Input: dimensioned drawing with shaded views. Units: mm. Origin: part minimum x, y, z. A direction names the side the tool comes from. Round coordinates to 2 decimals unless told otherwise and drop trailing zeros. Loops run counter-clockwise (first coordinate to the right, second up) from the corner with the lowest first, then second, coordinate; pieces in that order, holes last. Notation, with made-up numbers: (19, 18.5) - (74, 18.5) arc R21 cw to (74, 43.5) - close; hole circle Ø10 at (48, -10.75). An arc over 180 degrees is marked (long way). Use CSV: the item, a comma, the result in double quotes. Start each with the question number.
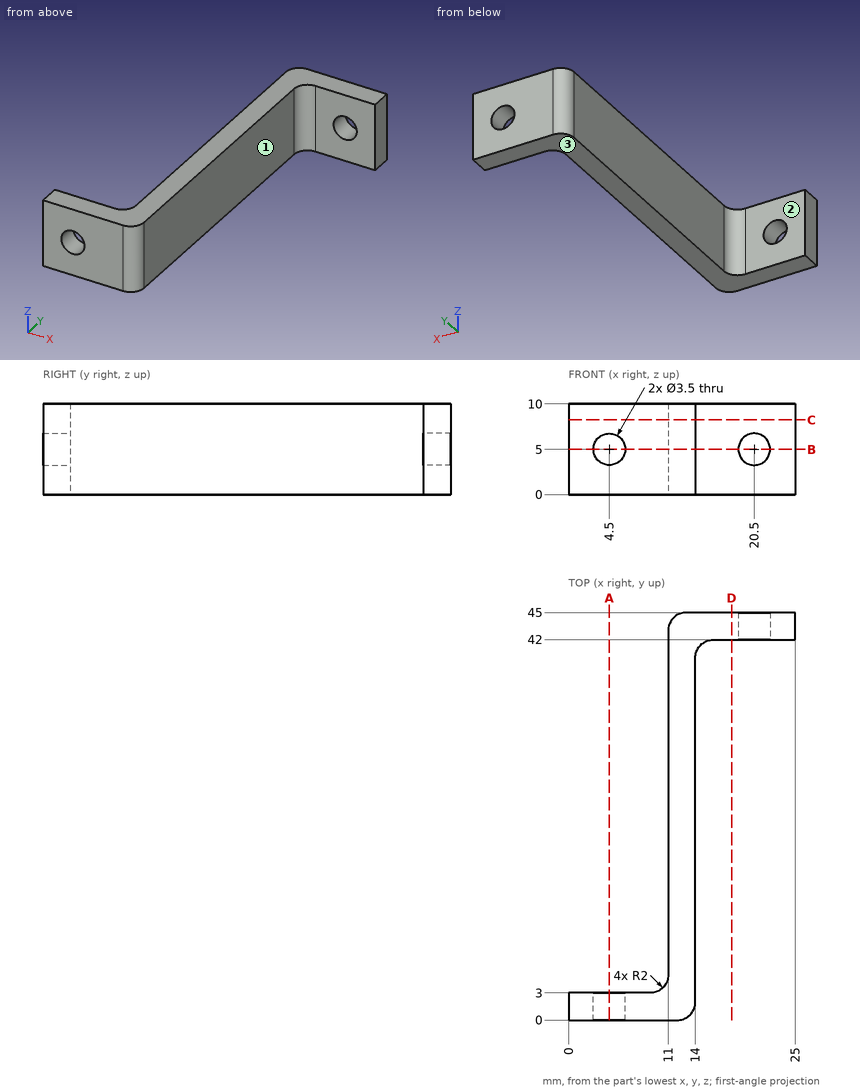
1. Section query B-B on z = 5. Return the cut outline in (x, y), and give its area (3 significant figures).
2. Contact query for flat-ended pins moving along their axis: P1, Ø5, axis at y = 11.5, z = 1, coming from the +X side; P2, Ø4.5, axis at x = 21.5, z = 6, coming from the -Y side; P3, Ø6, axis at y = 12.5, z = 7.5, coming from the -X side; P4, Ø5.5, axis at x = 4.5, z = 5, coming from the -Y side. Output: stop coordinate, or through.
3. Line query: line 1 along Z through (x, y) = (20.5, 44.25); line 2 along X through (y, z) = (2.2, 5); line 3 along X through (y, z) = (43, 5). Output: solid intervals per line, ascending.
4. Section query D-D on x = 18. Return the cut outline in (y, z), and give its area (3 significant figures).
5. Reachability of the marked faces 1, 2 and 3 from +Z, -Z, +X, -X, +Y, -Y: full face, straight path, thin tool, end or side. Return the list, or none.
6. Section query C-C on z = 8.25. Return the cut outline in (x, y), and give its area (3 significant figures).
7. Section query A-A on x = 4.5. Return the cut outline in (y, z).
Values:
1,outline,"(0, 0) - (2.75, 0) - (2.75, 3) - (0, 3) - close; (6.25, 0) - (12, 0) arc R2 ccw to (14, 2) - (14, 40) arc R2 cw to (16, 42) - (18.75, 42) - (18.75, 45) - (13, 45) arc R2 ccw to (11, 43) - (11, 5) arc R2 cw to (9, 3) - (6.25, 3) - close; (22.25, 42) - (25, 42) - (25, 45) - (22.25, 45) - close"
1,area,"180 mm^2"
2,P1,"stops at x = 14"
2,P2,"stops at y = 42"
2,P3,"stops at x = 11"
2,P4,"stops at y = 0"
3,line 1,"z = 0 to 3.25, 6.75 to 10"
3,line 2,"x = 0 to 2.75, 6.25 to 14"
3,line 3,"x = 11 to 18.75, 22.25 to 25"
4,outline,"(42, 0) - (45, 0) - (45, 10) - (42, 10) - close"
4,area,"30.0 mm^2"
5,face 1,"+Z, -Z, +X, -Y"
5,face 2,"+Z, -Z, -X, +Y"
5,face 3,"-Z, +X, -X, +Y, -Y"
6,outline,"(0, 0) - (12, 0) arc R2 ccw to (14, 2) - (14, 40) arc R2 cw to (16, 42) - (25, 42) - (25, 45) - (13, 45) arc R2 ccw to (11, 43) - (11, 5) arc R2 cw to (9, 3) - (0, 3) - close"
6,area,"201 mm^2"
7,outline,"(0, 0) - (3, 0) - (3, 3.25) - (0, 3.25) - close; (0, 6.75) - (3, 6.75) - (3, 10) - (0, 10) - close"
